```python
from build123d import *

# Parameters (mm, degrees)
SKETCH1_W           = 30
SKETCH1_H           = 56
SKETCH1_W_2         = 18
SKETCH1_H_2         = 51
SKETCH1_R           = 8.5
BOSS_EXTRUDE1_DEPTH = 2
SKETCH2_W           = 30
SKETCH2_H           = 56
SKETCH2_W_2         = 18
SKETCH2_H_2         = 44
BOSS_EXTRUDE2_DEPTH = 5
FILLET1_R           = 9
FILLET3_R           = 3
CHAMFER3_SIZE       = 5
SKETCH4_W           = 22.39143934
SKETCH4_H           = 45.199999578
BOSS_EXTRUDE3_DEPTH = 38.218999496
SKETCH5_W           = 15.39
SKETCH5_H           = 13.400000422
BOSS_EXTRUDE4_DEPTH = 2.6
FILLET4_R           = 5


with BuildPart() as part:
    # Sketch1 → Boss-Extrude1 (new body)
    # profile 1 of 2: a face of its own
    with BuildSketch(Plane.XY):
        with Locations((1.276e-06, 13.160000211)):
            Rectangle(SKETCH1_W, SKETCH1_H)
        with Locations((1.276e-06, 13.160000211)):
            Rectangle(SKETCH1_W_2, SKETCH1_H_2, mode=Mode.SUBTRACT)
    # profile 2 of 2: a face of its own
    with BuildSketch(Plane.XY):
        with Locations((1.276e-06, 13.160000211)):
            Rectangle(SKETCH1_W_2, SKETCH1_H_2)
        with Locations((1.276e-06, 26.160000211)):
            Circle(SKETCH1_R, mode=Mode.SUBTRACT)
        with Locations((1.276e-06, 0.160000211)):
            Circle(SKETCH1_R, mode=Mode.SUBTRACT)
    extrude(amount=-BOSS_EXTRUDE1_DEPTH)

    # Sketch2 → Boss-Extrude2 (add)
    with BuildSketch(Plane.XY):
        with Locations((1.276e-06, 13.160000211)):
            Rectangle(SKETCH2_W, SKETCH2_H)
        with Locations((1.276e-06, 13.160000211)):
            Rectangle(SKETCH2_W_2, SKETCH2_H_2, mode=Mode.SUBTRACT)
    extrude(amount=BOSS_EXTRUDE2_DEPTH)

    # Fillet1
    fillet1_edges = [part.edges().sort_by_distance(p)[0] for p in [
        (-14.999998724, -14.839999789, 1.5),
        (-14.999998724, 41.160000211, 1.5),
        (15.000001276, 41.160000211, 1.5),
        (15.000001276, -14.839999789, 1.5),
    ]]
    fillet(fillet1_edges, radius=FILLET1_R)

    # Fillet3
    fillet3_edges = [part.edges().sort_by_distance(p)[0] for p in [
        (-8.999998724, -8.839999789, 2.5),
        (9.000001276, -8.839999789, 2.5),
        (9.000001276, 35.160000211, 2.5),
        (-8.999998724, 35.160000211, 2.5),
    ]]
    fillet(fillet3_edges, radius=FILLET3_R)

    # Chamfer3
    chamfer3_edges = [part.edges().sort_by_distance(p)[0] for p in [
        (9.000001276, 13.160000211, 5),
        (8.121321619, 34.281320554, 5),
        (8.121321619, -7.961320133, 5),
        (-8.121319068, 34.281320554, 5),
        (-8.121319068, -7.961320133, 5),
        (-8.999998724, 13.160000211, 5),
        (1.276e-06, 35.160000211, 5),
        (1.276e-06, -8.839999789, 5),
    ]]
    chamfer(chamfer3_edges, length=CHAMFER3_SIZE - 0.0001)  # a hair under: the kernel refuses the full size

    # Sketch4 → Boss-Extrude3 (add)
    with BuildSketch(Plane(origin=(0, 0, -2), x_dir=(-1, 0, 0), z_dir=(0, 0, -1))):
        with BuildLine():
            Line((5.999998724, 41.160000211), (-6.000001276, 41.160000211))
            ThreePointArc((-6.000001276, 41.160000211), (-12.363962306, 38.523961242), (-15.000001276, 32.160000211))
            Line((-15.000001276, 32.160000211), (-15.000001276, -5.839999789))
            ThreePointArc((-15.000001276, -5.839999789), (-12.363962306, -12.20396082), (-6.000001276, -14.839999789))
            Line((-6.000001276, -14.839999789), (5.999998724, -14.839999789))
            ThreePointArc((5.999998724, -14.839999789), (12.363959755, -12.20396082), (14.999998724, -5.839999789))
            Line((14.999998724, -5.839999789), (14.999998724, 32.160000211))
            ThreePointArc((14.999998724, 32.160000211), (12.363959755, 38.523961242), (5.999998724, 41.160000211))
        make_face()
        with Locations((-0.84571967, 13.160000211)):
            Rectangle(SKETCH4_W, SKETCH4_H, mode=Mode.SUBTRACT)
    extrude(amount=BOSS_EXTRUDE3_DEPTH)

    # Sketch5 → Boss-Extrude4 (add)
    with BuildSketch(Plane(origin=(0, 0, -40.218999496), x_dir=(-1, 0, 0), z_dir=(0, 0, -1))):
        with BuildLine():
            Line((14.999998724, -5.839999789), (14.999998724, 32.160000211))
            ThreePointArc((14.999998724, 32.160000211), (12.363959755, 38.523961242), (5.999998724, 41.160000211))
            Line((5.999998724, 41.160000211), (-6.000001276, 41.160000211))
            ThreePointArc((-6.000001276, 41.160000211), (-12.363962306, 38.523961242), (-15.000001276, 32.160000211))
            Line((-15.000001276, 32.160000211), (-15.000001276, -5.839999789))
            ThreePointArc((-15.000001276, -5.839999789), (-12.363962306, -12.20396082), (-6.000001276, -14.839999789))
            Line((-6.000001276, -14.839999789), (5.999998724, -14.839999789))
            ThreePointArc((5.999998724, -14.839999789), (12.363959755, -12.20396082), (14.999998724, -5.839999789))
        make_face()
        with Locations((-1.845, 13.160000211)):
            Rectangle(SKETCH5_W, SKETCH5_H, mode=Mode.SUBTRACT)
    extrude(amount=-BOSS_EXTRUDE4_DEPTH)

    # Fillet4
    fillet4_edges = [part.edges().sort_by_distance(p)[0] for p in [
        (-14.999998724, 13.160000211, -40.218999496),
        (-12.363959755, 38.523961242, -40.218999496),
        (1.276e-06, 41.160000211, -40.218999496),
        (12.363962306, 38.523961242, -40.218999496),
        (15.000001276, 13.160000211, -40.218999496),
        (12.363962306, -12.20396082, -40.218999496),
        (1.276e-06, -14.839999789, -40.218999496),
        (-12.363959755, -12.20396082, -40.218999496),
    ]]
    fillet(fillet4_edges, radius=FILLET4_R)


solid = part.part
```
Could you check a few things on this model? Use its own coordinates, in mm. A direction names the side the tool comes from. Round coordinates to 2 decimals unless told otherwise and drop trailing zeros. Write each loop counter-clockwise with the first axis right and the second up, starting at its lowest first coordinate (ties: lowest second). Pieces come first, ordered by that corner, then holes.
(1) Suppose I cut it at A-A on z = -20. Write out the boundary of the cut face in (x, y).
Findings below:
outline: (-15, -5.84) arc R9 ccw to (-6, -14.84) - (6, -14.84) arc R9 ccw to (15, -5.84) - (15, 32.16) arc R9 ccw to (6, 41.16) - (-6, 41.16) arc R9 ccw to (-15, 32.16) - close; hole (-10.35, -9.44) - (12.04, -9.44) - (12.04, 35.76) - (-10.35, 35.76) - close
(2) Suppose I cut it at B-B on x = -4.5. State how many separate pieces and enclosed holes the cut face has, and give its area (3 significant figures).
Findings below:
separate pieces: 3
enclosed holes: 0
area: 574 mm2
(3) Which directions (+Z, -Z, +X, -X, +Y, -Y) give clear straight access to the entire face, cutting with the end or side of a thin tool? Please do faces 1 (the face through (0, 13, 0)), 2 (the face through (1, 35.76, -20)), 3 (the face through (2, 19.86, -39)).
Findings below:
face 1: +Z
face 2: none
face 3: -Z
(4) Thinking about a two-plate mould opening in X: for faces 4 (the face through (9.822, -9.747, 2.465)), 5 (the face through (-15, 13, -15)), 6 (the face through (-7, 13, -40.219)), 7 (the face through (-6.5, 13.5, -37.619)), which applies, +X half, -X half, draft (parallel to the pull), parting line (faces both ways), or undercut?
Findings below:
face 4: undercut
face 5: -X half
face 6: draft
face 7: undercut
(5) For pin 1 (0.8 mm diameter, centred on x = 2.5, z = -38.5, fed in from -Y); pin 2 (3 mm diameter, centred on x = -0.5, z = -39, fed in from +Y); pin 3 (0.8 mm diameter, centred on y = 15, z = -39.5, fed in from +X), each with a flat end and sliding along its axis, tell me the tip position at first contact or that it passes through.
Findings below:
pin 1: stops at y = -13.93
pin 2: stops at y = 40.61
pin 3: stops at x = 13.15
(6) Suppose I cut it at D-D on z = 1.5. Write out the boundary of the cut face in (x, y), and give its area (3 significant figures).
Findings below:
outline: (-15, -5.84) arc R9 ccw to (-6, -14.84) - (6, -14.84) arc R9 ccw to (15, -5.84) - (15, 32.16) arc R9 ccw to (6, 41.16) - (-6, 41.16) arc R9 ccw to (-15, 32.16) - close; hole (-10.5, -5.84) arc R4.5 ccw to (-6, -10.34) - (6, -10.34) arc R4.5 ccw to (10.5, -5.84) - (10.5, 32.16) arc R4.5 ccw to (6, 36.66) - (-6, 36.66) arc R4.5 ccw to (-10.5, 32.16) - close
area: 641 mm2
(7) If I drill on probe 1 along X at (y, z) = (10.5, -29.5); probe 2 along Y at (x, z) = (-2.5, -33.5); probe 3 along X at (y, z) = (0, -1), over which ranges is the centre line in solid material (lowest first)?
Findings below:
probe 1: x = -15 to -10.35, 12.04 to 15
probe 2: y = -14.84 to -9.44, 35.76 to 41.16
probe 3: x = -15 to -8.5, 8.5 to 15
